Read the model definition and answer for the solid it produces. Units are mm, in the model's axes. A direction names the side the tool comes from. Coordinates: 2 decimals unless noted, no trailing zeros. Order: outer loops, then holes, each group sorted by start corner. A loop starts at its lowest first (then second) coordinate and runs counter-clockwise, first axis right, second up.
Autodesk Inventor part; units mm, degrees
ref_plane "YZ Plane" through (0, 0, 0) normal (1, 0, 0) x (0, 1, 0)
ref_plane "XZ Plane" through (0, 0, 0) normal (0, 1, 0) x (-1, 0, 0)
ref_plane "XY Plane" through (0, 0, 0) normal (0, 0, 1) x (1, 0, 0)
sketch "Sketch1" plane through (0, 0, 0) normal (0, 1, 0) x (-1, 0, 0)
  line L0 (-1.27, -1.27) -> (1.27, -1.27)
  line L1 (1.27, -1.27) -> (1.27, 1.27)
  line L2 (1.27, 1.27) -> (-1.27, 1.27)
  line L3 (-1.27, 1.27) -> (-1.27, -1.27)
  line L4 (-1.27, -1.27) -> (1.27, 1.27) construction
  line L5 (1.27, -1.27) -> (-1.27, 1.27) construction
  point P0 (0, 0)
  dimension "d0" = 2.54
  dimension "d1" = 2.54
extrude "Extrusion1" add sketch "Sketch1" along normal blind 8.5
sketch "Sketch2" plane through (0, 8.5, 0) normal (0, 1, 0) x (1, 0, 0)
  circle A0 centre (0, 0) radius 0.35
  dimension "d4" = 0.7
extrude "Extrusion2" cut sketch "Sketch2" against normal blind 6
sketch "Sketch3" plane through (0, 0, 0) normal (0, -1, 0) x (1, 0, 0)
  circle A0 centre (0, 0) radius 0.325
  dimension "d7" = 0.65
extrude "Extrusion3" add sketch "Sketch3" along normal blind 6
properties part number "pin-header-female" material "Aluminum"
1) Straight lines are drawn through the part: line 1 (Z direction, x = 0, y = 4.2); line 2 (Y direction, x = 0.45, z = -0.2). For each, find the intervals that lie inside material, in ascending order.
A:
line 1: z = -1.27 to -0.35, 0.35 to 1.27
line 2: y = 0 to 8.5
2) A cutting plane is placed at D-D, the plane x = -0.8. Determine the outline of the cut face in (y, z), and give its area (3 significant figures).
A:
outline: (0, -1.27) - (8.5, -1.27) - (8.5, 1.27) - (0, 1.27) - close
area: 21.6 mm2
3) A cutting plane is placed at C-C, the plane z = 0. Determine the outline of the cut face in (x, y) (3 decimals), and give its area (3 significant figures).
A:
outline: (-1.27, 0) - (-0.325, 0) - (-0.325, -6) - (0.325, -6) - (0.325, 0) - (1.27, 0) - (1.27, 8.5) - (0.35, 8.5) - (0.35, 2.5) - (-0.35, 2.5) - (-0.35, 8.5) - (-1.27, 8.5) - close
area: 21.3 mm2
4) A flat-ended cylindrical pin translates along its axis: pin 1 Ø0.6 at (x, z) = (0, 0) entering from +Y. Find the tip coordinate at first contact, or state that the pin passes through.
A:
pin 1: stops at y = 2.5
5) A cutting plane is placed at A-A, the plane y = 4.5. Determine the outline of the cut face in (x, z).
A:
outline: (-1.27, -1.27) - (1.27, -1.27) - (1.27, 1.27) - (-1.27, 1.27) - close; hole circle Ø0.7 at (0, 0)
6) Which of the six approach directions +Z, -Z, +X, -X, +Y, -Y give full straight-line access (tool end or side, diameter ignored) to faces 1 (the flat face through (-1, 0, 0)), 2 (the flat face through (0, 4, 1.27))?
A:
face 1: -Y
face 2: +Z, +X, -X, +Y, -Y
7) A cutting plane is placed at B-B, the plane x = 0. Determine the outline of the cut face in (y, z) (3 decimals), and give its area (3 significant figures).
A:
outline: (-6, -0.325) - (0, -0.325) - (0, -1.27) - (8.5, -1.27) - (8.5, -0.35) - (2.5, -0.35) - (2.5, 0.35) - (8.5, 0.35) - (8.5, 1.27) - (0, 1.27) - (0, 0.325) - (-6, 0.325) - close
area: 21.3 mm2
